from build123d import *

# Parameters (mm, degrees)
SKETCH1_W                 = 13.5
SKETCH1_H                 = 2
SKETCH2_R                 = 5
BOSS_EXTRUDE1_DEPTH       = 0.3
SKETCH3_R                 = 4
BOSS_EXTRUDE2_DEPTH       = 2.2
SKETCH4_R                 = 5
BOSS_EXTRUDE3_DEPTH       = 0.5
F_8_CLEARANCE_HOLE1_D     = 4.5
F_8_CLEARANCE_HOLE1_DEPTH = 2.5
F_1_CLEARANCE_HOLE1_D     = 2.05
F_1_CLEARANCE_HOLE1_DEPTH = 2.5
F_2_CLEARANCE_HOLE1_D     = 2.5
F_2_CLEARANCE_HOLE1_DEPTH = 5
CHAMFER1_SIZE             = 0.325
CHAMFER2_SIZE2            = 0.200001177
CHAMFER2_SIZE             = 0.200001151
CHAMFER3_SIZE             = 0.2


with BuildPart() as part:
    # Sketch1 → Revolve1 (revolve)
    with BuildSketch(Plane(origin=(0, 0, 0), x_dir=(1, 0, 0), z_dir=(0, 1, 0))):
        with Locations((6.75, -1)):
            Rectangle(SKETCH1_W, SKETCH1_H)
    revolve(axis=Axis((0, 0, 0), (0, 0, 1)))

    # Sketch2 → Boss-Extrude1 (add)
    with BuildSketch(Plane.XY.offset(2)):
        Circle(SKETCH2_R)
    extrude(amount=BOSS_EXTRUDE1_DEPTH)

    # Sketch3 → Boss-Extrude2 (add)
    with BuildSketch(Plane.XY.offset(2.3)):
        Circle(SKETCH3_R)
    extrude(amount=BOSS_EXTRUDE2_DEPTH)

    # Sketch4 → Boss-Extrude3 (add)
    with BuildSketch(Plane(origin=(0, 0, 0), x_dir=(-1, 0, 0), z_dir=(0, 0, -1))):
        Circle(SKETCH4_R)
    extrude(amount=BOSS_EXTRUDE3_DEPTH)

    # #8 Clearance Hole1
    with Locations(Plane.XY.offset(2)):
        with Locations((3.061467459, 7.39103626), (7.39103626, 3.061467459), (7.39103626, -3.061467459), (3.061467459, -7.39103626), (-3.061467459, -7.39103626), (-7.39103626, -3.061467459), (-7.39103626, 3.061467459), (-3.061467459, 7.39103626)):
            Hole(F_8_CLEARANCE_HOLE1_D / 2, depth=F_8_CLEARANCE_HOLE1_DEPTH)

    # #1 Clearance Hole1
    with Locations(Plane.XY.offset(2)):
        with Locations((7.778174593, 7.778174593), (11, 0), (7.778174593, -7.778174593), (0, -11), (-7.778174593, -7.778174593), (-11, 0), (-7.778174593, 7.778174593), (0, 11)):
            Hole(F_1_CLEARANCE_HOLE1_D / 2, depth=F_1_CLEARANCE_HOLE1_DEPTH)

    # #2 Clearance Hole1
    with Locations(Plane.XY.offset(4.5)):
        with Locations((0, 0)):
            Hole(F_2_CLEARANCE_HOLE1_D / 2, depth=F_2_CLEARANCE_HOLE1_DEPTH)

    # Chamfer1
    chamfer1_edges = [part.edges().sort_by_distance(p)[0] for p in [
        (-6.753174593, -7.778174593, 2),
        (1.025, -11, 2),
        (8.803174593, -7.778174593, 2),
        (12.025, 0, 2),
        (8.803174593, 7.778174593, 2),
        (1.25, 0, 4.5),
        (1.025, 11, 2),
        (-6.753174593, 7.778174593, 2),
        (-9.975, 0, 2),
    ]]
    chamfer(chamfer1_edges, length=CHAMFER1_SIZE)

    # Chamfer2
    chamfer2_edges = [part.edges().sort_by_distance(p)[0] for p in [
        (-13.5, 0, 2),
        (-13.5, 0, 0),
    ]]
    chamfer(chamfer2_edges, length=CHAMFER2_SIZE, length2=CHAMFER2_SIZE2)

    # Chamfer3
    chamfer3_edges = [part.edges().sort_by_distance(p)[0] for p in [
        (-4, 0, 4.5),
        (5, 0, -0.5),
    ]]
    chamfer(chamfer3_edges, length=CHAMFER3_SIZE)


solid = part.part
Verification items for the finished model (mm, model axes). A direction names the side the tool comes from. Coordinates: 2 decimals unless noted, no trailing zeros. Order: outer loops, then holes, each group sorted by start corner. A loop starts at its lowest first (then second) coordinate and runs counter-clockwise, first axis right, second up. Notation, with made-up numbers: (45.5, 41) -> (49.5, 41) arc R31 cw to (49.5, 67) -> close; hole circle Ø1 at (75, -30.5). An arc over 180 degrees is marked (long way). Put each result on its own line as item: value. Start each with the question number.
1. Material ranges on L1, parallel to Y at x = 0, z = 1.25 (3 decimals); L2, parallel to Y at x = 0, z = 3.65; L3, parallel to Y at x = 4.5, z = 0.15, recorded low to high. Write a range as [from, to].
2. Mould release check, pull along Y, two halves, no side actions. Record for faces 1 (the flat face through (-1, -1, -0.5)), 2 (the cylindrical face through (3.549, 5.195, 0.986)), 3 (the cylindrical face through (-2.93, -13.18, 0.99)): released by +Y, released by -Y, zero draft, split by the parting line, or undercut.
3. Go/stop test with flat-tipped pins: pin 1 Ø8 at (x, y) = (-6, -7) entering from -Z; pin 2 Ø1.2 at (x, y) = (7.78, -7.78) entering from -Z; pin 3 Ø2.5 at (x, y) = (-7.78, 7.78) entering from +Z; pin 4 Ø5 at (x, y) = (-3.06, -7.39) entering from +Z. Record where each tip stops, or that it passes through.
4. Cross-section at C-C, the plane z = 3.1. Record the boundary of the cut face in (x, y), then the cut area to 3 significant figures.
5. Access from +Z, -Z, +X, -X, +Y, -Y to the whole of each face (thin tool, end or side, straight path). Record for faces 4 (the cylindrical face through (-0.867, -3.905, 3.286)), 5 (the cylindrical face through (-9.976, 0.045, 0.826)), 6 (the cylindrical face through (1.08, -4.88, -0.15)).
6. Cross-section at A-A, the plane z = 1. Count the separate pieces of the cut face and the enclosed holes in it, then the cut area to 3 significant figures.
Computed:
1. L1: [-13.5, -12.025], [-9.975, -1.25], [1.25, 9.975], [12.025, 13.5]
1. L2: [-4, -1.25], [1.25, 4]
1. L3: [-12.67, -9.12], [-5.66, 5.66], [9.12, 12.67]
2. face 1: zero draft
2. face 2: undercut
2. face 3: split by the parting line
3. pin 1: z = 0
3. pin 2: through
3. pin 3: z = 1.9
3. pin 4: z = 2
4. outline: circle Ø8 at (0, 0); hole circle Ø2.5 at (0, 0)
4. area: 45.4 mm2
5. face 4: +Z
5. face 5: +Z, -Z
5. face 6: -Z
6. separate pieces: 1
6. enclosed holes: 17
6. area: 414 mm2
